from build123d import *

# Parameters (mm, degrees)
F1_DEPTH = 11
F3_DEPTH = 11
F9_DEPTH = 4


with BuildPart() as f1:
    # F0 (on Right) → F1 (new body)
    with BuildSketch(Plane.YZ):
        with BuildLine():
            Line((-38, 0), (0, 0))
            Line((0, 0), (0, 38))
            ThreePointArc((0, 38), (-5.5649711575, 51.4350288425), (-19, 57))
            ThreePointArc((-19, 57), (-32.4350288425, 51.4350288425), (-38, 38))
            Line((-38, 38), (-38, 0))
        make_face()
    extrude(amount=F1_DEPTH)

    # F2 (on Top) → F3 (join)
    with BuildSketch(Plane.XY):
        with BuildLine():
            Line((38, 0), (0, 0))
            Line((0, 0), (0, -38))
            Line((0, -38), (38, -38))
            ThreePointArc((38, -38), (51.4350288425, -32.4350288425), (57, -19))
            ThreePointArc((57, -19), (51.4350288425, -5.5649711575), (38, 0))
        make_face()
    extrude(amount=F3_DEPTH)

    # F8 (on 3pt) → F9 (join, symmetric)
    with BuildSketch(Plane(origin=(0, -19, 0), x_dir=(-1, 0, 0), z_dir=(0, 1, 0))):
        Polygon((-11, 49), (-49, 11), (-11, 11), align=None)
    extrude(amount=F9_DEPTH, both=True)


solid = f1.part
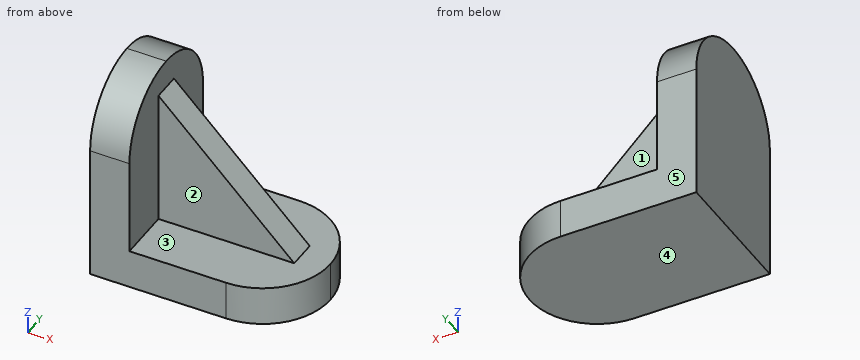
Design review of the part built by this model. Coordinates are the model's own, in mm. Face numbers are marked on the shaded views. A direction names the side the tool comes from. Round coordinates to 2 decimals unless told otherwise and drop trailing zeros. Loops run counter-clockwise (first coordinate to the right, second up) from the corner with the lowest first, then second, coordinate; pieces in that order, holes last. Notation, with made-up numbers: (-21.5, -37) - (0.5, -37) arc R17 ccw to (0.5, -32) - close; hole circle Ø8 at (29.5, 21.25). An arc over 180 degrees is marked (long way). One line per item, written item: value. Start each with the question number.
1) For the marked faces 1, 2, 3, 4 and 5, list the 3-axis set-ups (+Z, -Z, +X, -X, +Y, -Y) from which the entire face can be reached by the end or side of a thin tool; tool diameter is ignored.
2) Consider section B-B on x = 25. Give the boundary of the cut face in (y, z), then the cut area to 3 significant figures.
3) Insertion check: pin 1 Ø19 at (x, z) = (22, 23) entering from +Y; pin 2 Ø1 at (x, z) = (23, 31.5) entering from -Y; pin 3 Ø5 at (x, y) = (10, -27) entering from +Z. Each pin has a flat end and moves straight along its axis. Give the tip position at first contact, or say it passes through.
4) Consider section D-D on y = -5. Give the boundary of the cut face in (x, z), then the cut area to 3 significant figures.
5) Consider section C-C on y = -34.5. Give the boundary of the cut face in (x, z), then the cut area to 3 significant figures.
6) Consider section A-A on z = 34. Give the boundary of the cut face in (x, y), then the cut area to 3 significant figures.
7) To check wall thickness, follow L1, parallel to X at y = -34, z = 17; L2, parallel to Y at x = 13.5, z = 14. State the ranges of each line that lie inside material, in increasing order. Write a range as from..to.
Reported:
1. face 1: +Z, +X, +Y
1. face 2: +Z, +X, -Y
1. face 3: +Z, +X
1. face 4: -Z, +X, -X, +Y, -Y
1. face 5: +Z, -Z, +X, -X, +Y
2. outline: (-38, 0) - (0, 0) - (0, 11) - (-15, 11) - (-15, 35) - (-23, 35) - (-23, 11) - (-38, 11) - close
2. area: 610 mm^2
3. pin 1: stops at y = -15
3. pin 2: stops at y = -23
3. pin 3: stops at z = 56.19
4. outline: (0, 0) - (50.85, 0) - (50.85, 11) - (11, 11) - (11, 50.85) - (0, 50.85) - close
4. area: 998 mm^2
5. outline: (0, 0) - (48.99, 0) - (48.99, 11) - (11, 11) - (11, 48.99) - (0, 48.99) - close
5. area: 957 mm^2
6. outline: (0, -38) - (11, -38) - (11, -23) - (26, -23) - (26, -15) - (11, -15) - (11, 0) - (0, 0) - close
6. area: 538 mm^2
7. L1: x = 0..11
7. L2: y = -23..-15
